Autodesk Inventor part; units mm, degrees
ref_plane "YZ Plane" through (0, 0, 0) normal (1, 0, 0) x (0, 1, 0)
ref_plane "XZ Plane" through (0, 0, 0) normal (0, 1, 0) x (-1, 0, 0)
ref_plane "XY Plane" through (0, 0, 0) normal (0, 0, 1) x (1, 0, 0)
sketch "Sketch1" plane through (0, 0, 0) normal (0, 1, 0) x (-1, 0, 0)
  circle A0 centre (0, 0) radius 135
  circle A1 centre (0, 0) radius 110
  line L0 (0, 0) -> (-125, 0)
  line L1 (0, 0) -> (125, 0) construction
  circle A2 centre (-125, 0) radius 2.75
  circle A3 centre (-125, 0) radius 5
  dimension "d0" = 270
  dimension "d1" = 220
  dimension "d82" = 125
  dimension "d83" = 180
  dimension "d84" = 5.5
  dimension "d85" = 10
extrude "Extrusion1" add sketch "Sketch1" along normal mid plane 20 contours A0 | A2 | A3
sketch "Sketch4" plane through (0, 10, 0) normal (0, 1, 0) x (1, 0, 0)
  circle A0 centre (0, 0) radius 50.125
  circle A1 centre (0, 0) radius 135
  circle A2 centre (0, 0) radius 110
  line L0 (125.3494, 50.125) -> (150.3494, 50.125)
  line L1 (150.3494, 50.125) -> (150.3494, 35.125)
  line L2 (150.3494, 35.125) -> (125.3494, 35.125)
  line L3 (125.3494, 35.125) -> (125.3494, 50.125)
  line L4 (150.3494, 70.125) -> (104.7795, 70.125)
  line L5 (104.7795, 70.125) -> (104.7795, 85.125)
  line L6 (104.7795, 85.125) -> (150.3494, 85.125)
  line L7 (150.3494, 85.125) -> (150.3494, 70.125)
  line L8 (103.1497, 60.125) -> (138.3886, 60.125) construction
  point P0 (130.3504, 35.125)
  point P1 (115.3581, 70.125)
  dimension "d21" = 100.25
  dimension "d22" = 25
  dimension "d23" = 15
  dimension "d24" = 20
  dimension "d25" = 15
  dimension "d57" = 10
extrude "Extrusion3" add sketch "Sketch4" against normal up to surface (20 mm away) contours L6 L7 L4 A1 | A1 L0 L1 L2
fillet "Fillet1" radius 6 4 edges at (150.3494, 10, -77.625) (150.3494, -10, -77.625) (150.3494, -10, -42.625) (150.3494, 10, -42.625)
fillet "Fillet2" radius 10 1 edges at (104.7795, 0, -85.125)
fillet "Fillet3" radius 2 1 edges at (130.3504, 0, -35.125)
sketch "Sketch5" plane through (150.3494, -4, -85.125) normal (0, 0, -1) x (-1, 0, 0)
  line L0 (0, 8) -> (0, 0)
  line L1 (40.9135, -6) -> (6, -6)
  point P0 (150.3494, 4)
  point P1 (8, 4)
  point P2 (0, 4)
  dimension "d38" = 8
  dimension "d39" = 10
hole "Hole2" at (142.3494, 0, -85.125) direction (0, 0, 1) diameter 5 depth 50 counterbore diameter 8.5 counterbore depth 5
mirror "Mirror1" about plane through (0, 0, 0) normal (1, 0, 0) of "Extrusion3", "Fillet1", "Fillet2", "Fillet3", "Hole2"
mirror "Mirror2" about plane through (0, 0, 0) normal (0, 0, 1) of "Extrusion3", "Fillet1", "Fillet2", "Fillet3", "Hole2"
sketch "Sketch10" plane through (0, 10, 0) normal (0, 1, 0) x (1, 0, 0)
  line L0 (144.3494, 50.125) -> (125.3494, 50.125)
  line L1 (144.3494, -50.125) -> (125.3494, -50.125)
  line L2 (174.7146, 50.125) -> (75.699, 50.125)
  line L3 (75.699, 50.125) -> (75.699, -50.125)
  line L4 (75.699, -50.125) -> (174.7146, -50.125)
  line L5 (174.7146, 145.3293) -> (-157.7861, 145.3293)
  line L6 (-157.7861, 145.3293) -> (-157.7861, -141.1771)
  line L7 (-157.7861, -141.1771) -> (174.7146, -141.1771)
  line L8 (174.7146, -141.1771) -> (174.7146, -50.125)
  line L9 (174.7146, 50.125) -> (174.7146, 145.3293)
  point P0 (0, 0)
extrude "Extrusion7" cut sketch "Sketch10" against normal through all
fillet "Fillet7" radius 2 2 edges at (97.9157, 0, -50.125) (97.9157, 0, 50.125)
sketch "Sketch12" plane through (0, 10, 0) normal (0, 1, 0) x (1, 0, 0)
  circle A0 centre (0, 0) radius 110
  line L0 (122.5, 30) -> (97.5, 30)
  line L1 (97.5, 30) -> (97.5, -30)
  line L2 (97.5, -30) -> (122.5, -30)
  line L3 (122.5, -30) -> (122.5, 30)
  line L4 (122.5, 30) -> (97.5, -30) construction
  line L5 (97.5, 30) -> (122.5, -30) construction
  point P0 (110, 0)
  dimension "d68" = 25
  dimension "d69" = 60
extrude "Extrusion9" cut sketch "Sketch12" against normal up to surface (20 mm away) contours A0 L2 L1 L0 | A0 L0 L3 L2 picked at (101.6667, 0)
fillet "Fillet8" radius 8 2 edges at (122.5, 0, -30) (122.5, 0, 30)
extrude "Extrusion10" cut sketch "Sketch1" along normal mid plane 20 contours A2 | A3
extrude "Extrusion11" add sketch "Sketch1" along normal up to surface (10 mm away) contours A3
properties part number "Cylinder 80-20 Spacer_1 Slant"
The listing builds one solid part. Answer for the finished solid, in the listing's coordinates (mm). A direction names the side the tool comes from. Coordinates: 2 decimals unless noted, no trailing zeros. Write each loop counter-clockwise with the first axis right and the second up, starting at its lowest first coordinate (ties: lowest second). Pieces come first, ordered by that corner, then holes.
Q1. Section B-B, the plane y = 1.5 is taken. Give the number of separate pieces and of enclosed holes in the cut face, then the cut area to 3 significant figures.
Returned:
separate pieces: 3
enclosed holes: 1
area: 2,320 mm2
Q2. Given P1, Ø2, axis at y = 0.5, z = -11, coming from the -X side; P2, Ø4.5, axis at x = 142.35, y = 0, coming from the +Z side; P3, Ø8, axis at x = 125, z = 0, coming from the -Y side, each flat-ended and moving along its own axis, determine where each tip first touches the part or whether it passes through.
Returned:
P1: stops at x = 122.5
P2: passes through
P3: stops at y = 0
Q3. Section D-D, the plane x = 125 is taken. Write down the section's boundary in (y, z) (3 decimals).
Returned:
outline: (-10, -50.125) - (10, -50.125) - (10, -2.75) - (0, -2.75) - (0, -5) - (-10, -5) - close; (-10, 5) - (0, 5) - (0, 2.75) - (10, 2.75) - (10, 50.125) - (-10, 50.125) - close
Q4. The mould has two halves that part along Y. Classify faces 1 (the flat face through (122, 10, 1)), 2 (the cylindrical face through (102.896, -0.14, -38.89)), 3 (the cylindrical face through (144.57, 1.15, -42.52)): released by +Y, released by -Y, zero draft, split by the parting line, or undercut.
Returned:
face 1: released by +Y
face 2: zero draft
face 3: undercut
Q5. Find the intervals of material crossed by line 1 along Z through (x, y) = (125, 7.75) (3 decimals); line 2 along Z through (x, y) = (135.5, 5.5) (3 decimals); line 3 along X through (y, z) = (5.25, -2), in increasing order.
Returned:
line 1: z = -50.125 to -2.75, 2.75 to 50.125
line 2: z = -50.125 to -35.125, 35.125 to 50.125
line 3: x = 120.42 to 123.11, 126.89 to 134.99
Q6. Which of the six approach directions +Z, -Z, +X, -X, +Y, -Y give full straight-line access (tool end or side, diameter ignored) to faces 4 (the cylindrical face through (102.987, -0.14, 38.648)), 5 (the flat face through (122.8, 0, -2.2)), 6 (the flat face through (140, 2, -35.125))?
Returned:
face 4: -X, +Y, -Y
face 5: -Y
face 6: +X, +Y, -Y
Q7. Section A-A, the plane x = 111.5 is taken. Write down the section's boundary in (y, z) (3 decimals).
Returned:
outline: (-10, -50.125) - (10, -50.125) - (10, -30) - (-10, -30) - close; (-10, 30) - (10, 30) - (10, 50.125) - (-10, 50.125) - close
